Geometry check sheet. Reference: the model listing, model coordinates, mm. A direction names the side the tool comes from. Round coordinates to 2 decimals unless told otherwise and drop trailing zeros. Order: outer loops, then holes, each group sorted by start corner. A loop starts at its lowest first (then second) coordinate and runs counter-clockwise, first axis right, second up.
(1) Sectioned sample at B-B (y = 17.78). Record the boundary of the cut face in (x, z), plus the area to 3 significant figures.
(2) Set-up check for faces 3 (the face through (0, 5.08, 38)), 4 (the face through (-13.927, 2.504, 22.45)): record each of +Z, -Z, +X, -X, +Y, -Y from which the full face is reachable in a straight line by a thin tool's end or side.
(3) Sectioned sample at D-D (x = 0). Record the boundary of the cut face in (y, z), plus the area to 3 significant figures.
(4) Go/stop test with flat-tipped pins: pin 1 (6.5 mm diameter, centred on x = -22.5, z = 38.1, fed in from +Y); pin 2 (3 mm diameter, centred on x = 0, z = 60.6, fed in from -Y); pin 3 (5 mm diameter, centred on x = -8, z = 30.5, fed in from -Y). Record where each tip stops, or that it passes through.
(5) Material ranges on line 1 along X through (y, z) = (3, 38); line 2 along Y through (x, z) = (35.95, 19.05); line 3 along X through (y, z) = (20, 11), recorded low to high.
(6) Sectioned sample at A-A (z = 38.1). Record the boundary of the cut face in (x, y), plus the area to 3 significant figures.
(7) Release check for a two-part mould opening along X. For faces 1 (the face through (35.52, 32.2, 17.17)), 2 (the face through (-33.02, 21, 38)) record: +X half, -X half, draft (parallel to the pull), parting line (faces both ways), or undercut.
(8) Sectioned sample at C-C (x = 22.5). Record the boundary of the cut face in (y, z).
from build123d import *

# Parameters (mm, degrees)
BOSS_EXTRUDE1_DEPTH = 76.2
FILLET1_R           = 1.6
SKETCH2_R           = 2
CUT_EXTRUDE2_DEPTH  = 93.814324864
SKETCH3_R           = 2.55
CUT_EXTRUDE3_DEPTH  = 114.882961412


with BuildPart() as part:
    # Sketch1 → Boss-Extrude1 (new body)
    with BuildSketch(Plane.XY):
        Polygon((-38.1, 0), (38.1, 0), (38.1, 3.175), (38.1, 36.83), (33.02, 36.83), (33.02, 5.08), (-33.02, 5.08), (-33.02, 36.83), (-38.1, 36.83), (-38.1, 4.389392044), align=None)
    extrude(amount=BOSS_EXTRUDE1_DEPTH)

    # Fillet1
    fillet1_edges = [part.edges().sort_by_distance(p)[0] for p in [
        (-33.02, 36.83, 38.1),
        (-33.02, 5.08, 38.1),
        (33.02, 5.08, 38.1),
        (33.02, 36.83, 38.1),
    ]]
    fillet(fillet1_edges, radius=FILLET1_R)

    # Sketch2 → Cut-Extrude2 (cut, through all)
    with BuildSketch(Plane.XZ):
        with Locations(Location((0, 60.6, 0), (0, 0, 270))):
            Circle(SKETCH2_R)
        with Locations(Location((15.909902577, 54.009902577, 0), (0, 0, 270))):
            Circle(SKETCH2_R)
        with Locations(Location((22.5, 38.1, 0), (0, 0, 270))):
            Circle(SKETCH2_R)
        with Locations(Location((15.909902577, 22.190097423, 0), (0, 0, 270))):
            Circle(SKETCH2_R)
        with Locations(Location((0, 15.6, 0), (0, 0, 270))):
            Circle(SKETCH2_R)
        with Locations(Location((-15.909902577, 22.190097423, 0), (0, 0, 270))):
            Circle(SKETCH2_R)
        with Locations(Location((-22.5, 38.1, 0), (0, 0, 270))):
            Circle(SKETCH2_R)
        with Locations(Location((-15.909902577, 54.009902577, 0), (0, 0, 270))):
            Circle(SKETCH2_R)
    extrude(amount=-CUT_EXTRUDE2_DEPTH, mode=Mode.SUBTRACT)

    # Sketch3 → Cut-Extrude3 (cut, through all)
    with BuildSketch(Plane.ZY.offset(38.1)):
        with Locations((19.05, 30.48)):
            Circle(SKETCH3_R)
        with Locations((19.05, 17.78)):
            Circle(SKETCH3_R)
        with Locations((57.15, 17.78)):
            Circle(SKETCH3_R)
        with Locations((57.15, 30.48)):
            Circle(SKETCH3_R)
    extrude(amount=-CUT_EXTRUDE3_DEPTH, mode=Mode.SUBTRACT)


solid = part.part
Answer below:
1. outline: (-38.1, 0) - (-33.02, 0) - (-33.02, 16.5) - (-38.1, 16.5) - close; (-38.1, 21.6) - (-33.02, 21.6) - (-33.02, 54.6) - (-38.1, 54.6) - close; (-38.1, 59.7) - (-33.02, 59.7) - (-33.02, 76.2) - (-38.1, 76.2) - close; (33.02, 0) - (38.1, 0) - (38.1, 16.5) - (33.02, 16.5) - close; (33.02, 21.6) - (38.1, 21.6) - (38.1, 54.6) - (33.02, 54.6) - close; (33.02, 59.7) - (38.1, 59.7) - (38.1, 76.2) - (33.02, 76.2) - close
1. area: 671 mm2
2. face 3: +Z, -Z, +Y
2. face 4: +Y, -Y
3. outline: (0, 0) - (5.08, 0) - (5.08, 13.6) - (0, 13.6) - close; (0, 17.6) - (5.08, 17.6) - (5.08, 58.6) - (0, 58.6) - close; (0, 62.6) - (5.08, 62.6) - (5.08, 76.2) - (0, 76.2) - close
3. area: 346 mm2
4. pin 1: stops at y = 5.08
4. pin 2: passes through
4. pin 3: stops at y = 0
5. line 1: x = -38.1 to -24.5, -20.5 to 20.5, 24.5 to 38.1
5. line 2: y = 0 to 15.23, 20.33 to 27.93, 33.03 to 36.83
5. line 3: x = -38.1 to -33.02, 33.02 to 38.1
6. outline: (-38.1, 0) - (-24.5, 0) - (-24.5, 5.08) - (-31.42, 5.08) arc R1.6 cw to (-33.02, 6.68) - (-33.02, 35.23) arc R1.6 ccw to (-34.62, 36.83) - (-38.1, 36.83) - close; (-20.5, 0) - (20.5, 0) - (20.5, 5.08) - (-20.5, 5.08) - close; (24.5, 0) - (38.1, 0) - (38.1, 36.83) - (34.62, 36.83) arc R1.6 ccw to (33.02, 35.23) - (33.02, 6.68) arc R1.6 cw to (31.42, 5.08) - (24.5, 5.08) - close
6. area: 669 mm2
7. face 1: draft
7. face 2: undercut
8. outline: (0, 0) - (5.08, 0) - (5.08, 36.1) - (0, 36.1) - close; (0, 40.1) - (5.08, 40.1) - (5.08, 76.2) - (0, 76.2) - close
